Job drawing, mm, ordinate dimensions from the low corner. One solid piece. A direction names the side the tool comes from. Give positions to 0.01 mm unless a question says otherwise; leave off trailing zeros. Loops run counter-clockwise (first coordinate to the right, second up) from the corner with the lowest first, then second, coordinate; pieces in that order, holes last. Notation, with made-up numbers: M 37.5,84 L 77.5,84 A14 ccw 77.5,101 Z; hole C 22.25,84 d9. An arc over 180 degrees is marked long. Answer in a Markdown table with one row per item.
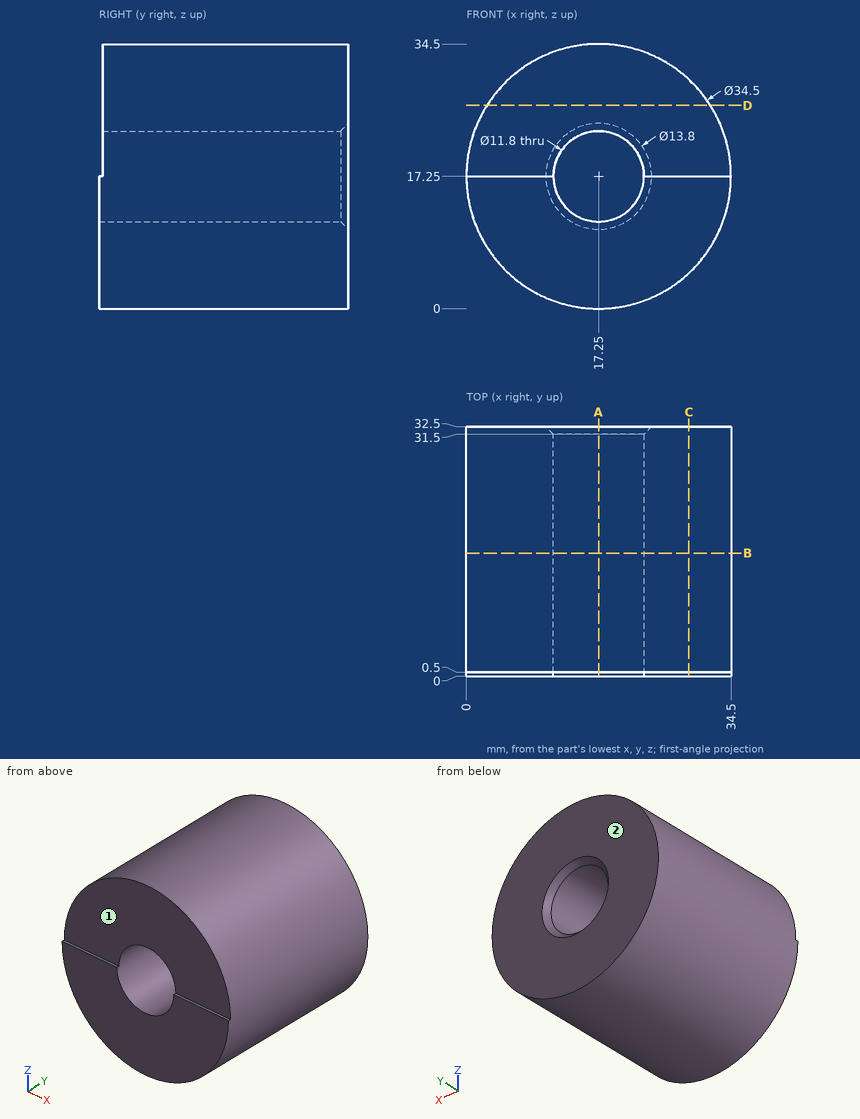
(1) Drill centre lines: line 1 along X through (y, z) = (18, 17.25); line 2 along Y through (x, z) = (24.5, 26). Where is each one in solid material? Low to high.
Recorded:
| item | result |
|---|---|
| line 1 | x = 0 to 11.35, 23.15 to 34.5 |
| line 2 | y = 0.5 to 32.5 |
(2) Saw through at B-B (y = 16). Write the cut outline in (x, z).
Recorded:
| item | result |
|---|---|
| outline | C 17.25,17.25 d34.5; hole C 17.25,17.25 d11.8 |
(3) Saw through at D-D (z = 26.5). Write the cut outline in (x, y), plus the area to 3 significant figures.
Recorded:
| item | result |
|---|---|
| outline | M 2.69,0.5 L 31.81,0.5 L 31.81,32.5 L 2.69,32.5 Z |
| area | 932 mm^2 |
(4) Saw through at A-A (x = 17.25). Write the cut outline in (y, z), plus the area to 3 significant figures.
Recorded:
| item | result |
|---|---|
| outline | M 0,0 L 32.5,0 L 32.5,10.35 L 31.5,11.35 L 0,11.35 Z; M 0.5,23.15 L 31.5,23.15 L 32.5,24.15 L 32.5,34.5 L 0.5,34.5 Z |
| area | 731 mm^2 |
(5) Which spindle directions (+Z, -Z, +X, -X, +Y, -Y) get a long thin tool onto all of the face, cutting with end or side? Do the marked faces 1 and 2. Say none if no direction does.
Recorded:
| item | result |
|---|---|
| face 1 | +Z, +X, -X, -Y |
| face 2 | +Z, -Z, +X, -X, +Y |
(6) Pin check, flat tips, straight feed: pin 1 Ø1 at (x, y) = (31, 17) entering from +Z; pin 2 Ø4 at (y, z) = (6, 23) entering from -X; pin 3 Ø4 at (x, y) = (3.5, 21.5) entering from +Z. Stop position of each tip, or through.
Recorded:
| item | result |
|---|---|
| pin 1 | stops at z = 28.3 |
| pin 2 | stops at x = 0.41 |
| pin 3 | stops at z = 29.88 |
(7) Saw through at C-C (x = 29). Write the cut outline in (y, z), plus the area to 3 significant figures.
Recorded:
| item | result |
|---|---|
| outline | M 0,4.62 L 32.5,4.62 L 32.5,29.88 L 0.5,29.88 L 0.5,17.25 L 0,17.25 Z |
| area | 815 mm^2 |
